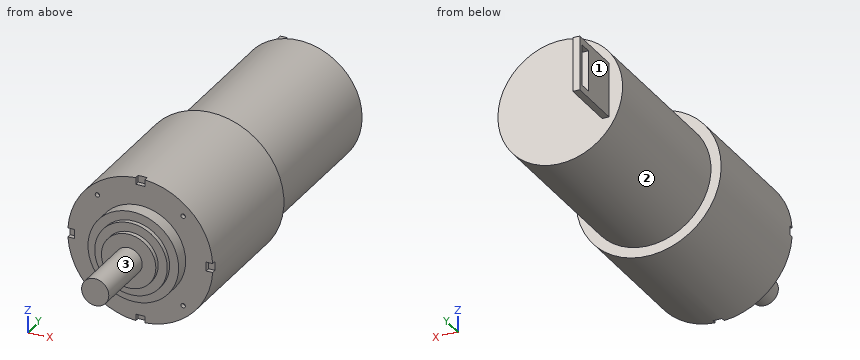
Autodesk Inventor part; units mm, degrees
ref_plane "YZ Plane" through (0, 0, 0) normal (1, 0, 0) x (0, 1, 0)
ref_plane "XZ Plane" through (0, 0, 0) normal (0, 1, 0) x (-1, 0, 0)
ref_plane "XY Plane" through (0, 0, 0) normal (0, 0, 1) x (1, 0, 0)
sketch "Sketch1" plane through (0, 0, 0) normal (0, 1, 0) x (-1, 0, 0)
  circle A0 centre (0, 0) radius 16
  dimension "d0" = 32
extrude "Extrusion1" add sketch "Sketch1" along normal blind 30.4
sketch "Sketch2" plane through (0, 30.4, 0) normal (0, 1, 0) x (1, 0, 0)
  circle A0 centre (0, 0) radius 13.75
  dimension "d3" = 27.5
extrude "Extrusion2" add sketch "Sketch2" along normal blind 37.8
sketch "Sketch3" plane through (0, 0, 0) normal (0, -1, 0) x (1, 0, 0)
  circle A0 centre (0, 0) radius 10
  dimension "d6" = 20
extrude "Extrusion3" add sketch "Sketch3" along normal blind 3
sketch "Sketch4" plane through (0, -3, 0) normal (0, -1, 0) x (1, 0, 0)
  circle A0 centre (0, 0) radius 8
  dimension "d9" = 16
extrude "Extrusion4" add sketch "Sketch4" along normal blind 1
sketch "Sketch5" plane through (0, -4, 0) normal (0, -1, 0) x (1, 0, 0)
  circle A0 centre (0, 0) radius 6
  dimension "d12" = 12
extrude "Extrusion5" add sketch "Sketch5" along normal blind 1
sketch "Sketch6" plane through (0, -5, 0) normal (0, -1, 0) x (1, 0, 0)
  circle A0 centre (0, 0) radius 3
  dimension "d15" = 6
extrude "Extrusion6" add sketch "Sketch6" along normal blind 14.3
sketch "Sketch7" plane through (0, 68.2, 0) normal (0, 1, 0) x (1, 0, 0)
  line L0 (-9.25, -6) -> (-10.75, -6)
  line L1 (-10.75, -6) -> (-10.75, 6)
  line L2 (-10.75, 6) -> (-9.25, 6)
  line L3 (-9.25, 6) -> (-9.25, -6)
  circle A0 centre (0, 0) radius 10
  line L4 (-9.25, -6) -> (-10.75, 6) construction
  line L5 (-10.75, -6) -> (-9.25, 6) construction
  point P0 (-10, 0)
  dimension "d18" = 12
  dimension "d19" = 1.5
extrude "Extrusion7" add sketch "Sketch7" along normal blind 12.5 contours L0 L1 L2 L3 A0 | A0 L3 picked at (-9.4369, 0.6455)
sketch "Sketch8" plane through (-10.75, 68.2, -6) normal (-1, 0, 0) x (0, 0, 1)
  line L0 (1.5, 11.5) -> (10.5, 11.5)
  line L1 (10.5, 11.5) -> (10.5, 8.812)
  line L2 (10.5, 8.812) -> (1.5, 8.812)
  line L3 (1.5, 8.812) -> (1.5, 11.5)
  line L4 (0, 12.5) -> (12, 12.5)
  line L5 (0, 0) -> (0, 12.5)
  line L6 (12, 0) -> (12, 12.5)
  point P0 (6, -68.2)
  dimension "d22" = 1
  dimension "d23" = 1.5
  dimension "d24" = 1.5
extrude "Extrusion8" cut sketch "Sketch8" against normal through all
sketch "Sketch9" plane through (0, 0, 0) normal (0, -1, 0) x (1, 0, 0)
  circle A0 centre (0, 0) radius 13.75
  line L0 (-9.4443, 9.9933) -> (9.4443, 9.9933)
  line L1 (9.4443, 9.9933) -> (9.4443, -9.9933)
  line L2 (9.4443, -9.9933) -> (-9.4443, -9.9933)
  line L3 (-9.4443, -9.9933) -> (-9.4443, 9.9933)
  line L4 (-9.4443, 9.9933) -> (9.4443, -9.9933) construction
  line L5 (9.4443, 9.9933) -> (-9.4443, -9.9933) construction
  circle A1 centre (9.4443, -9.9933) radius 0.5
  circle A2 centre (-9.4443, -9.9933) radius 0.5
  circle A3 centre (-9.4443, 9.9933) radius 0.5
  circle A4 centre (9.4443, 9.9933) radius 0.5
  dimension "d27" = 1
  dimension "d28" = 1
  dimension "d29" = 1
  dimension "d30" = 1
extrude "Extrusion9" cut sketch "Sketch9" against normal blind 1 contours A4 L1 A0 | A0 A4 | A1 A0 | A0 L1 A1 | L0 A4 A0 | L1 A4 L0 | L2 A1 L1 | A0 A1 L2 | A3 L0 A0 | A0 A3 | A3 L3 L0 | A2 A0 | A0 L2 A2 | L2 L3 A2 | L3 A3 A0 | A0 A2 L3
sketch "Sketch10" plane through (0, 0, 0) normal (0, -1, 0) x (1, 0, 0)
  circle A0 centre (0, 0) radius 16
  line L0 (0, 16) -> (0, 14.5)
  line L1 (0, 14.5) -> (-1, 14.5)
  line L2 (-1, 14.5) -> (-1, 16)
  line L3 (-1, 16) -> (0, 16)
  line L4 (0, 16) -> (0, 14.5)
  line L5 (0, 14.5) -> (1, 14.5)
  line L6 (1, 14.5) -> (1, 16)
  line L7 (1, 16) -> (0, 16)
  dimension "d33" = 1
  dimension "d34" = 1
  dimension "d35" = 1.5
extrude "Extrusion10" cut sketch "Sketch10" against normal blind 1 contours L6 L5 L0 A0 | A0 L7 L6 | L2 L3 A0 | A0 L0 L1 L2
mirror "Mirror1" about plane through (0, 0, 0) normal (0, 0, 1) of "Extrusion10"
sketch "Sketch11" plane through (0, 0, 0) normal (0, -1, 0) x (1, 0, 0)
  arc A0 (1, -15.9687) -> (1, 15.9687) centre (0, 0) ccw
  line L0 (16, 0) -> (14.5, 0)
  line L1 (14.5, 0) -> (14.5, 1)
  line L2 (14.5, 1) -> (16, 1)
  line L3 (16, 1) -> (16, 0)
  line L4 (16, 0) -> (14.5, 0)
  line L5 (14.5, 0) -> (14.5, -1)
  line L6 (14.5, -1) -> (16, -1)
  line L7 (16, -1) -> (16, 0)
  dimension "d38" = 1
  dimension "d39" = 1
  dimension "d40" = 1.5
extrude "Extrusion11" cut sketch "Sketch11" against normal blind 1
mirror "Mirror2" about plane through (0, 0, 0) normal (1, 0, 0) of "Extrusion11"
properties part number "CorrectMotor_CAD_spencermical_enes100OSVproject_4-50pm-3-3-16-thursday-freshmanyear-springsemester"
The listing builds one solid part. Answer for the finished solid, in the listing's coordinates (mm). Face numbers are marked on the shaded views. A direction names the side the tool comes from. Coordinates: 2 decimals unless noted, no trailing zeros. Write each loop counter-clockwise with the first axis right and the second up, starting at its lowest first coordinate (ties: lowest second). Pieces come first, ordered by that corner, then holes. Notation, with made-up numbers: M 85.5,-26.75 L 115.5,-26.75 A20 cw 115.5,-0.75 Z; hole C -27.75,59 d9. An arc over 180 degrees is marked long. Write each question's results on one line, items separated by ' | '.
Item 1: The part is cut by section C-C on x = 12. Determine the outline of the cut face in (y, z), and give its area (3 significant figures).
Answer below:
outline: M 0,-10.58 L 30.4,-10.58 L 30.4,-6.71 L 68.2,-6.71 L 68.2,6.71 L 30.4,6.71 L 30.4,10.58 L 0,10.58 Z | area: 1,150 mm2
Item 2: The part is cut by section B-B on y = 56. Determine the outline of the cut face in (x, z).
Answer below:
outline: C 0,0 d27.5
Item 3: Consider probe 1 along Y at (x, z) = (-2.5, 13); probe 2 along Z at (x, y) = (0, 51.5); probe 3 along Y at (x, z) = (-10, -11). Determine where each line is inside the solid, lowest interval first. Write a range as [from, to].
Answer below:
probe 1: [0, 68.2] | probe 2: [-13.75, 13.75] | probe 3: [0, 30.4]
Item 4: The part is cut by section A-A on x = 0. Determine the outline of the cut face in (y, z).
Answer below:
outline: M -19.3,-3 L -5,-3 L -5,-6 L -4,-6 L -4,-8 L -3,-8 L -3,-10 L 0,-10 L 0,-14.5 L 1,-14.5 L 1,-16 L 30.4,-16 L 30.4,-13.75 L 68.2,-13.75 L 68.2,13.75 L 30.4,13.75 L 30.4,16 L 1,16 L 1,14.5 L 0,14.5 L 0,10 L -3,10 L -3,8 L -4,8 L -4,6 L -5,6 L -5,3 L -19.3,3 Z
Item 5: Given P1, Ø4, axis at x = -9.5, y = 49.5, coming from the +Z side; P2, Ø1, axis at x = -0.5, y = 13, coming from the -Z side; P3, Ø8, axis at x = 2.5, z = -8, coming from the -Y side; P4, Ø1.1, axis at x = 15, y = 0.5, coming from the -Z side, each flat-ended and moving along its own axis, determine where each tip first touches the part or whether it passes through.
Answer below:
P1: z = 11.52 | P2: z = -16 | P3: y = -5 | P4: z = -6.87
Item 6: Which of the six approach directions +Z, -Z, +X, -X, +Y, -Y give full straight-line access (tool end or side, diameter ignored) to the marked faces 1, 2 and 3?
Answer below:
face 1: +Z, -Z, -X, +Y | face 2: +Y | face 3: -Y
